Can you work these out from the model? Positions are in its coordinate system, mm. Coordinates: 2 decimals unless noted, no trailing zeros. Order: outer loops, then holes, each group sorted by start corner. A loop starts at its lowest first (then second) coordinate and runs counter-clockwise, first axis right, second up.
```python
from build123d import *

# Parameters (mm, degrees)
SKETCH1_R            = 39
SKETCH1_R_2          = 26.5
BOSS_EXTRUDE1_DEPTH  = 1
SKETCH3_W            = 50
SKETCH3_H            = 51.5
BOSS_EXTRUDE2_DEPTH  = 1
BOSS_EXTRUDE3_DEPTH  = 1
BOSS_EXTRUDE5_DEPTH  = 1
SKETCH2_R            = 2.75
CUT_EXTRUDE1_DEPTH   = 2
CIRPATTERN1_COUNT    = 6
CUT_EXTRUDE2_START   = -3
SKETCH5_R            = 2.25
CUT_EXTRUDE2_DEPTH   = 4
LPATTERN1_COUNT      = 2
LPATTERN1_PITCH      = 15
LPATTERN1_COUNT_DIR2 = 2
LPATTERN1_PITCH_DIR2 = 10
LPATTERN2_COUNT      = 2
LPATTERN2_PITCH      = 15
LPATTERN2_COUNT_DIR2 = 2
LPATTERN2_PITCH_DIR2 = 10
CUT_EXTRUDE3_START   = -3
SKETCH8_R            = 4.25
CUT_EXTRUDE3_DEPTH   = 4
LPATTERN3_COUNT      = 3
LPATTERN3_PITCH      = 20


with BuildPart() as part:
    # Sketch1 → Boss-Extrude1 (new body, symmetric)
    with BuildSketch(Plane(origin=(0, 0, 0), x_dir=(1, 0, 0), z_dir=(0, 1, 0))):
        Circle(SKETCH1_R)
        Circle(SKETCH1_R_2, mode=Mode.SUBTRACT)
    extrude(amount=BOSS_EXTRUDE1_DEPTH, both=True)

    # Sketch3 → Boss-Extrude2 (add, symmetric)
    with BuildSketch(Plane(origin=(0, 0, 0), x_dir=(1, 0, 0), z_dir=(0, 1, 0))):
        with Locations((0, 52.25)):
            Rectangle(SKETCH3_W, SKETCH3_H)
    extrude(amount=BOSS_EXTRUDE2_DEPTH, both=True)

    # Sketch4 → Boss-Extrude3 (add, symmetric)
    with BuildSketch(Plane(origin=(0, 0, 0), x_dir=(1, 0, 0), z_dir=(0, 1, 0))):
        Polygon((-25, 53.966629547), (-37.466824315, 10.827607112), (-25, 29.933259094), align=None)
        Polygon((37.466824315, 10.827607112), (25, 29.933259094), (25, 53.966629547), align=None)
    extrude(amount=BOSS_EXTRUDE3_DEPTH, both=True)

    # Sketch7 → Boss-Extrude5 (add, symmetric)
    with BuildSketch(Plane(origin=(0, 0, 0), x_dir=(1, 0, 0), z_dir=(0, 1, 0))):
        Polygon((120, -40), (26.5, -40), (0, -39), (26.5, -15.728301656), (26.5, 0), (26.5, 40), (120, 40), align=None)
    extrude(amount=BOSS_EXTRUDE5_DEPTH, both=True)

    # Sketch2 → Cut-Extrude1 (cut, symmetric)
    with BuildSketch(Plane(origin=(0, 0, 0), x_dir=(1, 0, 0), z_dir=(0, 1, 0))):
        with Locations((0, 32.5)):
            Circle(SKETCH2_R)
    cut_extrude1 = extrude(amount=CUT_EXTRUDE1_DEPTH, both=True, mode=Mode.SUBTRACT)

    # CirPattern1: Cut-Extrude1 ×6 about axis
    cirpattern1_axis = Axis((0, 0, 0), (0, 1, 0))
    for i in range(1, CIRPATTERN1_COUNT):
        add(cut_extrude1.rotate(cirpattern1_axis, i * 360 / CIRPATTERN1_COUNT), mode=Mode.SUBTRACT)

    # Sketch5 → Cut-Extrude2 (cut)
    with BuildSketch(Plane(origin=(0, 1, 0), x_dir=(1, 0, 0), z_dir=(0, 1, 0)).offset(CUT_EXTRUDE2_START)):
        with Locations((0, 73)):
            Circle(SKETCH5_R)
    cut_extrude2 = extrude(amount=CUT_EXTRUDE2_DEPTH, mode=Mode.SUBTRACT)

    # LPattern1: Cut-Extrude2 2 × 2
    with Locations(*[(i * LPATTERN1_PITCH, 0, j * LPATTERN1_PITCH_DIR2) for i in range(LPATTERN1_COUNT) for j in range(LPATTERN1_COUNT_DIR2) if (i, j) != (0, 0)]):
        add(cut_extrude2, mode=Mode.SUBTRACT)

    # LPattern2: Cut-Extrude2 2 × 2
    with Locations(*[(-i * LPATTERN2_PITCH, 0, j * LPATTERN2_PITCH_DIR2) for i in range(LPATTERN2_COUNT) for j in range(LPATTERN2_COUNT_DIR2) if (i, j) != (0, 0)]):
        add(cut_extrude2, mode=Mode.SUBTRACT)

    # Sketch8 → Cut-Extrude3 (cut)
    with BuildSketch(Plane(origin=(0, 1, 0), x_dir=(1, 0, 0), z_dir=(0, 1, 0)).offset(CUT_EXTRUDE3_START)):
        with Locations((60, 20)):
            Circle(SKETCH8_R)
        with Locations((60, -20)):
            Circle(SKETCH8_R)
    cut_extrude3 = extrude(amount=CUT_EXTRUDE3_DEPTH, mode=Mode.SUBTRACT)

    # LPattern3: Cut-Extrude3 ×3
    with Locations(*[(i * LPATTERN3_PITCH, 0, 0) for i in range(1, LPATTERN3_COUNT)]):
        add(cut_extrude3, mode=Mode.SUBTRACT)


solid = part.part
```
1. Imagine slicing it at A-A on z = -73. Please give me the cut outline in (x, y).
Completed:
outline: (-25, -1) - (-17.25, -1) - (-17.25, 1) - (-25, 1) - close; (-12.75, -1) - (-2.25, -1) - (-2.25, 1) - (-12.75, 1) - close; (2.25, -1) - (12.75, -1) - (12.75, 1) - (2.25, 1) - close; (17.25, -1) - (25, -1) - (25, 1) - (17.25, 1) - close
2. Please list where these lines run through material, in increasing order: probe 1 along Z at (x, y) = (0, -0.6); probe 2 along X at (y, z) = (0.85, -21.5); probe 3 along Z at (x, y) = (77.5, 0.35).
Completed:
probe 1: z = -78 to -75.25, -70.75 to -65.25, -60.75 to -35.25, -29.75 to -26.5, 26.5 to 29.75, 35.25 to 39
probe 2: x = -34.38 to -15.49, 15.49 to 56.02, 63.98 to 76.02, 83.98 to 96.02, 103.98 to 120
probe 3: z = -40 to -23.44, -16.56 to 16.56, 23.44 to 40
3. I'm going to push flat-ended pins straight in: pin 1 (1 mm diameter, centred on x = 59.5, y = 0.5, fed in from -Z); pin 2 (0.6 mm diameter, centred on y = 0.5, z = -62.5, fed in from +X). Where does each tip first touch, or does it pass through?
Completed:
pin 1: stops at z = -40
pin 2: stops at x = 25
4. Imagine slicing it at C-C on z = -5. Please give me the cut outline in (x, y), then the cut area to 3 significant figures.
Completed:
outline: (-38.68, -1) - (-26.02, -1) - (-26.02, 1) - (-38.68, 1) - close; (26.02, -1) - (120, -1) - (120, 1) - (26.02, 1) - close
area: 213 mm2
5. Imagine slicing it at D-D on y = 0.4. Give the number of separate pieces and of enclosed holes in the cut face, then the cut area to 3 significant figures.
Completed:
separate pieces: 1
enclosed holes: 19
area: 11,300 mm2
6. Thinking about a two-plate mould opening in Z: for faces 1 (the flat face through (42, 1, -7)), 2 (the cylindrical face through (25.523, 0.014, -15.424)), 3 (the flat face through (26.99, 0.01, -47.08)), which applies, pulls with the +Z half, pulls with the -Z half, needs draft (parallel to the pull), parting line crosses it, or undercut?
Completed:
face 1: needs draft
face 2: undercut
face 3: pulls with the -Z half
7. Imagine slicing it at B-B on x = 100. Please give me the cut outline in (y, z).
Completed:
outline: (-1, -40) - (1, -40) - (1, -24.25) - (-1, -24.25) - close; (-1, -15.75) - (1, -15.75) - (1, 15.75) - (-1, 15.75) - close; (-1, 24.25) - (1, 24.25) - (1, 40) - (-1, 40) - close
